The listing builds one solid part. Answer for the finished solid, in the listing's coordinates (mm). A direction names the side the tool comes from. Round coordinates to 2 decimals unless told otherwise and drop trailing zeros. Loops run counter-clockwise (first coordinate to the right, second up) from the corner with the lowest first, then second, coordinate; pieces in that order, holes last. Notation, with made-up numbers: (-1, -15) -> (16, -15) arc R13 ccw to (16, -1) -> close; hole circle Ø9 at (12.5, -9.5). An arc over 180 degrees is marked (long way). One line per question, with ' | ' between items.
from build123d import *

# Parameters (mm, degrees)
SKETCH1_R           = 31.75
SKETCH1_R_2         = 14.2875
BOSS_EXTRUDE1_DEPTH = 4.7625
SKETCH1_3_R         = 2.25
BOSS_EXTRUDE2_DEPTH = 4.7625
SKETCH1_5_R         = 2.5
CUT_EXTRUDE1_DEPTH  = 5.7625
CIRPATTERN1_COUNT   = 6


with BuildPart() as part:
    # Sketch1 → Boss-Extrude1 (new body, symmetric)
    with BuildSketch(Plane.XY):
        Circle(SKETCH1_R)
        Circle(SKETCH1_R_2, mode=Mode.SUBTRACT)
    extrude(amount=BOSS_EXTRUDE1_DEPTH, both=True)

    # Sketch1_3 → Boss-Extrude2 (add, symmetric)
    with BuildSketch(Plane.XY):
        with BuildLine():
            ThreePointArc((-16.975976856, 103.864226407), (-10.380000805, 110.063559945), (-19.004913728, 112.811197739))
            ThreePointArc((-19.004913728, 112.811197739), (-43.981596647, 65.290659685), (-31.853644116, 12.993919882))
            ThreePointArc((-31.853644116, 12.993919882), (-30.783267014, 10.305575859), (-30.872393941, 7.4133523))
            ThreePointArc((-30.872393941, 7.4133523), (-27.701380897, 15.51438031), (-22.45064034, 22.450640265))
            ThreePointArc((-22.45064034, 22.450640265), (-28.712576811, 20.475279906), (-33.923533352, 24.470255355))
            ThreePointArc((-33.923533352, 24.470255355), (-40.260809011, 64.341772494), (-24.504598742, 101.512201327))
            ThreePointArc((-24.504598742, 101.512201327), (-21.096215477, 103.827506526), (-16.975976856, 103.864226407))
        make_face()
        with Locations((-15.5, 108.902479311)):
            Circle(SKETCH1_3_R, mode=Mode.SUBTRACT)
        with BuildLine():
            ThreePointArc((-20.572826284, 29.17582828), (-20.629600002, 25.566924084), (-22.45064034, 22.450640265))
            ThreePointArc((-22.45064034, 22.450640265), (-16.232909422, 27.286537921), (-9.016045552, 30.442953579))
            ThreePointArc((-9.016045552, 30.442953579), (-14.868295469, 31.271240847), (-18.073412893, 36.237337019))
            ThreePointArc((-18.073412893, 36.237337019), (-11.212505299, 76.061130888), (17.805097778, 104.185592177))
            ThreePointArc((17.805097778, 104.185592177), (18.158136201, 113.429819804), (10.257775708, 108.616849345))
            ThreePointArc((10.257775708, 108.616849345), (9.542205751, 105.099281948), (7.199837842, 102.379239056))
            ThreePointArc((7.199837842, 102.379239056), (-18.077740957, 70.099262208), (-20.572826284, 29.17582828))
        make_face()
        with Locations((15.5, 108.902479311)):
            Circle(SKETCH1_3_R, mode=Mode.SUBTRACT)
    boss_extrude2 = extrude(amount=BOSS_EXTRUDE2_DEPTH, both=True)

    # Sketch1_5 → Cut-Extrude1 (cut, symmetric)
    with BuildSketch(Plane.XY):
        with Locations((-20.622229928, 11.90625)):
            Circle(SKETCH1_5_R)
    cut_extrude1 = extrude(amount=CUT_EXTRUDE1_DEPTH, both=True, mode=Mode.SUBTRACT)

    # CirPattern1: Boss-Extrude2, Cut-Extrude1 ×6 about axis
    cirpattern1_axis = Axis((0, 0, 0), (0, 0, 1))
    for i in range(1, CIRPATTERN1_COUNT):
        add(boss_extrude2.rotate(cirpattern1_axis, i * 360 / CIRPATTERN1_COUNT))
        add(cut_extrude1.rotate(cirpattern1_axis, i * 360 / CIRPATTERN1_COUNT), mode=Mode.SUBTRACT)


solid = part.part
Q1. Given pin 1 Ø3 at (x, y) = (-20.62, 11.91) entering from +Z; pin 2 Ø1 at (x, z) = (-63.5, 1.5) entering from -Y; pin 3 Ø1.5 at (x, z) = (58.5, 1.5) entering from +Y; pin 4 Ø4 at (y, z) = (74, -1) entering from +X, each flat-ended and moving along its own axis, determine where each tip first touches the part or whether it passes through.
Numbers:
pin 1: through | pin 2: y = -76.68 | pin 3: y = 76.52 | pin 4: x = 89.81
Q2. A cutting plane is placed at B-B on y = 82. Give the vertices of the cut face in (x, z).
Numbers:
outline: (-39.89, -4.76) -> (-35.82, -4.76) -> (-35.82, 4.76) -> (-39.89, 4.76) -> close; (-12.2, -4.76) -> (-7.66, -4.76) -> (-7.66, 4.76) -> (-12.2, 4.76) -> close
Q3. A cutting plane is placed at C-C on z = -0.75. Give the number of separate pieces and of enclosed holes in the cut face, plus the area to 3 significant figures.
Numbers:
separate pieces: 1 | enclosed holes: 19 | area: 8,080 mm^2
Q4. For a pull along X with two mould halves and no side action, classify faces 1 (the face through (-8, 14, 4.762)), 2 (the face through (43.88, -66.05, 0.07)) as pulls with the +X half, pulls with the -X half, needs draft (parallel to the pull), parting line crosses it, or undercut.
Numbers:
face 1: needs draft | face 2: undercut
Q5. For faces 3 (the face through (95.84, 44.29, 0.07)), 4 (the face through (-11.48, 75.55, 0.07)), determine the directions among +Z, -Z, +X, -X, +Y, -Y from which every point of the face is accessible in a straight line to the end or side of a thin tool.
Numbers:
face 3: +Z, -Z, +Y | face 4: +Z, -Z
Q6. Find the intervals of material crossed by line 1 (Y direction, x = -72.5, z = -1.25); line 2 (Y direction, x = 0, z = -1); line 3 (Y direction, x = -28, z = -2.75), in increasing order. Write a range as from..to.
Numbers:
line 1: -76.24..-72.41, -50.9..-47.05, -9.61..-5.07, 23..30 | line 2: -96.66..-91.38, -42.17..-26.31, -21.31..-14.29, 14.29..21.31, 26.31..42.17, 91.38..96.66 | line 3: -67.63..-63.28, -42.22..-37.77, -21.13..20.39, 96.82..103.24
Q7. A cutting plane is placed at A-A on x = -49.5. Give the vertices of the cut face in (y, z).
Numbers:
outline: (-75.26, -4.76) -> (-71.38, -4.76) -> (-71.38, 4.76) -> (-75.26, 4.76) -> close; (-50.32, -4.76) -> (-46.43, -4.76) -> (-46.43, 4.76) -> (-50.32, 4.76) -> close; (-19.17, -4.76) -> (-15.25, -4.76) -> (-15.25, 4.76) -> (-19.17, 4.76) -> close; (2.54, -4.76) -> (6.93, -4.76) -> (6.93, 4.76) -> (2.54, 4.76) -> close
